Check sheet for the modelled part. Datum: model origin and axes. Units: mm. A direction names the side the tool comes from. Round coordinates to 2 decimals unless told otherwise and drop trailing zeros. Order: outer loops, then holes, each group sorted by start corner. A loop starts at its lowest first (then second) coordinate and runs counter-clockwise, first axis right, second up.
(1) Depth check by flat-ended pin: pin 1 (3 mm diameter, centred on y = 12.5, z = -27.5, fed in from -X) (3 decimals); pin 2 (7 mm diameter, centred on y = 9.525, z = -31.75, fed in from -X); pin 3 (4 mm diameter, centred on x = -12.7, y = 9.525, fed in from +Z); pin 4 (5 mm diameter, centred on y = 16.5, z = -16.5, fed in from +X). Enter the tip coordinate at first touch or a pass-through.
(2) Tool access check on faces 4 (the flat face through (-9, 9, -41.275)), 5 (the cylindrical face through (-0.45, 8.01, -14.36)). Record the directions out of +Z, -Z, +X, -X, +Y, -Y that give a thin tool (end or side, any length) a straight path to the whole face; none if there is none.
(3) Sectioned sample at D-D, the plane z = -21.5. Enter the section's corners in (x, y) (3 decimals).
(4) Sectioned sample at B-B, the plane x = -12.7. Enter the section's corners in (y, z) (3 decimals).
(5) Mould release check, pull along X, two halves, no side actions. Record for faces 1 (the cylindrical face through (-10.768, 12.045, -1.61)), 2 (the cylindrical face through (-0.449, 10.893, -33.534)), 3 (the flat face through (-3.175, 9, -22)): released by +X, released by -X, zero draft, split by the parting line, or undercut.
(6) Sectioned sample at C-C, the plane x = -6. Enter the section's corners in (y, z) (3 decimals), and give its area (3 significant figures).
(7) Thickness scan on probe 1 along Z at (x, y) = (-6.75, 3.5) (3 decimals); probe 2 along Y at (x, z) = (-0.5, -12.7); probe 3 along Y at (x, z) = (-12.7, -43.75). Record the ranges inside material, lowest first.
Autodesk Inventor part; units mm, degrees
ref_plane "YZ Plane" through (0, 0, 0) normal (1, 0, 0) x (0, 1, 0)
ref_plane "XZ Plane" through (0, 0, 0) normal (0, 1, 0) x (-1, 0, 0)
ref_plane "XY Plane" through (0, 0, 0) normal (0, 0, 1) x (1, 0, 0)
sketch "Sketch1" plane through (0, 0, 0) normal (0, 1, 0) x (-1, 0, 0)
  line L0 (0, 0) -> (19.05, 0)
  line L1 (19.05, 0) -> (19.05, -3.175)
  line L2 (19.05, -3.175) -> (0, -3.175)
  line L3 (0, -3.175) -> (0, 0)
  line L4 (0, 0) -> (3.175, 0)
  line L5 (3.175, 0) -> (3.175, -44.45)
  line L6 (3.175, -44.45) -> (0, -44.45)
  line L7 (0, -44.45) -> (0, 0)
  line L8 (0, -44.45) -> (19.05, -44.45)
  line L9 (19.05, -44.45) -> (19.05, -41.275)
  line L10 (19.05, -41.275) -> (0, -41.275)
  line L11 (0, -41.275) -> (0, -44.45)
  dimension "d0" = 19.05
  dimension "d1" = 3.175
  dimension "d2" = 3.175
  dimension "d3" = 44.45
  dimension "d4" = 19.05
  dimension "d5" = 3.175
extrude "Extrusion1" add sketch "Sketch1" along normal blind 19.05
sketch "Sketch2" plane through (-19.05, 0, 0) normal (0, 0, 1) x (1, 0, 0)
  line L0 (0, 0) -> (0, 19.05)
  line L1 (0, 0) -> (19.05, 0)
  line L2 (19.05, 0) -> (19.05, 19.05)
  point P0 (6.35, 9.525)
  dimension "d9" = 19.05
  dimension "d10" = 9.525
  dimension "d18" = 12.7
hole "Hole1" at (-12.7, 9.525, 0) direction (0, 0, -1) diameter 6.35 end through all
sketch "Sketch3" plane through (-3.175, 0, -41.275) normal (-1, 0, 0) x (0, 0, 1)
  line L0 (0, 19.05) -> (38.1, 19.05)
  line L1 (0, 0) -> (38.1, 0)
  line L2 (38.1, 0) -> (38.1, 19.05)
  line L3 (0, 0) -> (0, 19.05)
  point P0 (41.275, 0)
  point P1 (9.525, 9.525)
  point P2 (28.575, 9.525)
  dimension "d19" = 9.525
  dimension "d20" = 19.05
  dimension "d21" = 9.525
  dimension "d22" = 9.525
  dimension "d23" = 9.525
hole "Hole2" at (-3.175, 9.525, -31.75) at (-3.175, 9.525, -12.7) direction (1, 0, 0) diameter 4.4958 end through all countersink diameter 8.4328 countersink angle 82
equation "\"d4\" = d0"
properties part number "CAR_045_NewCarouselTensioner1.75UChannel" material "Aluminum 6061"
Derived:
1. pin 1: stops at x = -3.175
1. pin 2: stops at x = -2.35
1. pin 3: passes through
1. pin 4: stops at x = 0
2. face 4: -X, +Y, -Y
2. face 5: +X, -X
3. outline: (-3.175, 0) - (0, 0) - (0, 19.05) - (-3.175, 19.05) - close
4. outline: (0, -44.45) - (6.35, -44.45) - (6.35, -41.275) - (0, -41.275) - close; (0, -3.175) - (6.35, -3.175) - (6.35, 0) - (0, 0) - close; (12.7, -44.45) - (19.05, -44.45) - (19.05, -41.275) - (12.7, -41.275) - close; (12.7, -3.175) - (19.05, -3.175) - (19.05, 0) - (12.7, 0) - close
5. face 1: undercut
5. face 2: zero draft
5. face 3: released by -X
6. outline: (0, -44.45) - (19.05, -44.45) - (19.05, -41.275) - (0, -41.275) - close; (0, -3.175) - (19.05, -3.175) - (19.05, 0) - (0, 0) - close
6. area: 121 mm2
7. probe 1: z = -44.45 to -41.275, -3.175 to 0
7. probe 2: y = 0 to 7.28, 11.77 to 19.05
7. probe 3: y = 0 to 6.35, 12.7 to 19.05
